Answer from the drawing. Dimensions are ordinates in mm from the lowest x, y and z of the part. A direction names the side the tool comes from. Give positions to 0.01 mm unless a question says otherwise; leave off trailing zeros. Write each loop counter-clockwise with the first axis right and the second up, starting at its lowest first coordinate (ties: lowest second). Pieces come first, ordered by that corner, then holes. Notation, with made-up numbers: (31.25, 24.5) -> (62.25, 24.5) arc R34 ccw to (62.25, 60.5) -> close; hole circle Ø3 at (88.25, 5.5). An arc over 180 degrees is marked (long way). Use a Markdown table: item, result. Add a question column.
Q1. For the marked faces 1 and 2, determine the directions among +Z, -Z, +X, -X, +Y, -Y from which every point of the face is accessible in a straight line to the end or side of a thin tool.
Q2. Section B-B, the plane z = 19 is taken. Give the vertices of the cut face in (x, y).
Q3. Each of these flat-tipped pins is pushed along its axis until it touches: pin 1 Ø1.5 at (x, z) = (2, 11.5) entering from -Y; pin 2 Ø1 at (y, z) = (3.5, 16) entering from +X; pin 3 Ø1.5 at (x, z) = (1.5, 11) entering from +Y (1 decimal). Where does it stop, or does it pass through?
Q4. Section A-A, the plane z = 5 is taken. Give the vertices of the cut face in (x, y).
Q5. Consider line 1 (Z direction, x = 5.75, y = 3); line 2 (X direction, y = 3, z = 17); line 3 (X direction, y = 2.6, z = 8). Determine where each line is inside the solid, lowest interval first.
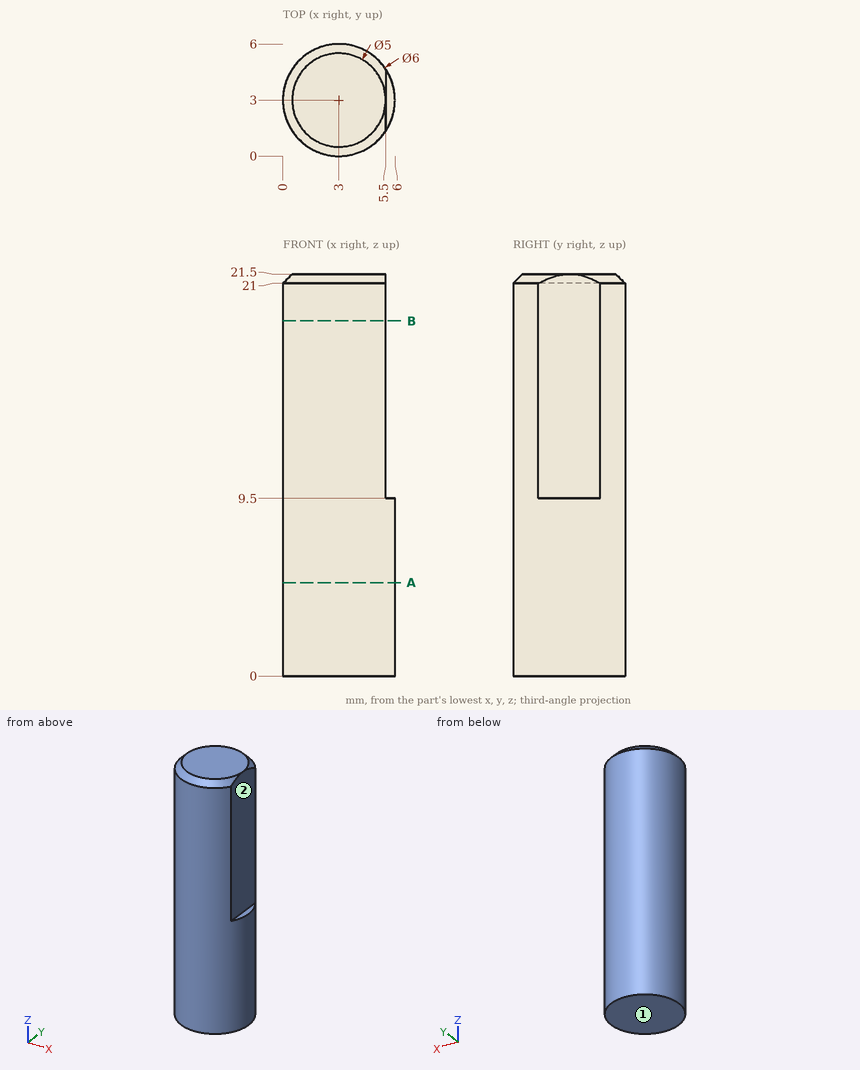
Result set:
| question | item | result |
|---|---|---|
| 1 | face 1 | -Z, +X, -X, +Y, -Y |
| 1 | face 2 | +Z, +X, +Y, -Y |
| 2 | outline | (5.5, 1.34) -> (5.5, 4.66) arc R3 ccw (long way) to start |
| 3 | pin 1 | stops at y = 0.01 |
| 3 | pin 2 | stops at x = 5.5 |
| 3 | pin 3 | stops at y = 5.9 |
| 4 | outline | circle Ø6 at (3, 3) |
| 5 | line 1 | z = 0 to 9.5 |
| 5 | line 2 | x = 0 to 5.5 |
| 5 | line 3 | x = 0.03 to 5.97 |
